Read the model definition and answer for the solid it produces. Units are mm, in the model's axes. Face numbers are marked on the shaded views. Coordinates: 2 decimals unless noted, no trailing zeros. Order: outer loops, then holes, each group sorted by start corner. A loop starts at its lowest first (then second) coordinate and runs counter-clockwise, first axis right, second up. Notation, with made-up numbers: (16.5, 84) -> (28.5, 84) arc R18 ccw to (28.5, 90) -> close; hole circle Ø6 at (-17, 89.5). An arc over 180 degrees is marked (long way). Answer in a Markdown table with one row per item.
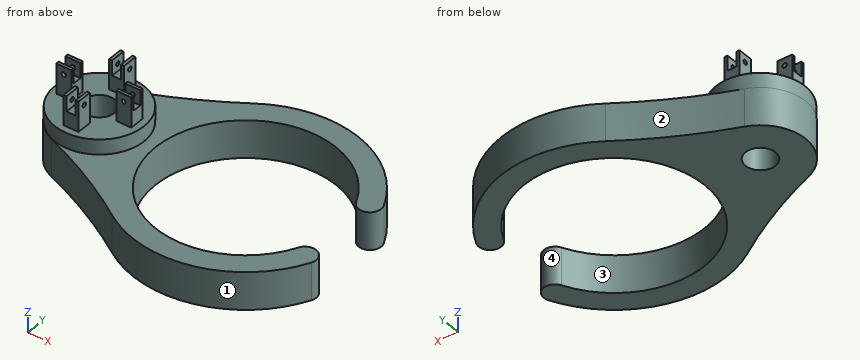
from build123d import *

# Parameters (mm, degrees)
BOSS_EXTRUDE1_DEPTH = 25
SKETCH1_3_R         = 29.652029199
BOSS_EXTRUDE2_DEPTH = 35
SKETCH3_R           = 10
CUT_EXTRUDE1_DEPTH  = 35
SKETCH4_W           = 10
SKETCH4_H           = 10
BOSS_EXTRUDE3_DEPTH = 20
SKETCH5_W           = 6
SKETCH5_H           = 10
SKETCH5_W_2         = 10
SKETCH5_H_2         = 6
CUT_EXTRUDE2_DEPTH  = 10
SKETCH6_R           = 1.3
SKETCH6_R_2         = 1.5
CUT_EXTRUDE3_DEPTH  = 10
SKETCH7_R           = 1.5
CUT_EXTRUDE4_DEPTH  = 10


with BuildPart() as part:
    # Sketch1 → Boss-Extrude1 (new body)
    with BuildSketch(Plane.XY):
        with BuildLine():
            ThreePointArc((50.600725893, 12.618751535), (112.455741461, 2.776716043), (160.210090254, 43.303630369))
            ThreePointArc((160.210090254, 43.303630369), (156.582418814, 53.270575735), (146.615473448, 49.642904296))
            ThreePointArc((146.615473448, 49.642904296), (32.237006226, 75), (146.615473448, 100.357095704))
            ThreePointArc((146.615473448, 100.357095704), (156.582418814, 96.729424265), (160.210090254, 106.696369631))
            ThreePointArc((160.210090254, 106.696369631), (112.455741461, 147.223283957), (50.600725893, 137.381248465))
            ThreePointArc((50.600725893, 137.381248465), (18.262261371, 118.334618782), (-16.010570265, 103.040064143))
            ThreePointArc((-16.010570265, 103.040064143), (-35.344980602, 75), (-16.010570265, 46.959935857))
            ThreePointArc((-16.010570265, 46.959935857), (18.262261371, 31.665381218), (50.600725893, 12.618751535))
        make_face()
    extrude(amount=BOSS_EXTRUDE1_DEPTH)

    # Sketch1<3> → Boss-Extrude2 (add)
    with BuildSketch(Plane.XY):
        with Locations((-5.344980602, 75)):
            Circle(SKETCH1_3_R)
    extrude(amount=BOSS_EXTRUDE2_DEPTH)

    # Sketch3 → Cut-Extrude1 (cut)
    with BuildSketch(Plane.XY.offset(35)):
        with Locations((-5.344980602, 75)):
            Circle(SKETCH3_R)
    extrude(amount=-CUT_EXTRUDE1_DEPTH, mode=Mode.SUBTRACT)

    # Sketch4 → Boss-Extrude3 (add)
    with BuildSketch(Plane.XY.offset(35)):
        with Locations((14.655019398, 75)):
            Rectangle(SKETCH4_W, SKETCH4_H)
        with Locations((-5.344980602, 55)):
            Rectangle(SKETCH4_W, SKETCH4_H)
        with Locations((-5.344980602, 95)):
            Rectangle(SKETCH4_W, SKETCH4_H)
        with Locations((-25.344980602, 75)):
            Rectangle(SKETCH4_W, SKETCH4_H)
    extrude(amount=BOSS_EXTRUDE3_DEPTH)

    # Sketch5 → Cut-Extrude2 (cut)
    with BuildSketch(Plane.XY.offset(55)):
        with Locations((-5.344980602, 95)):
            Rectangle(SKETCH5_W, SKETCH5_H)
        with Locations((14.655019398, 75)):
            Rectangle(SKETCH5_W_2, SKETCH5_H_2)
        with Locations((-5.344980602, 55)):
            Rectangle(SKETCH5_W, SKETCH5_H)
        with Locations((-25.344980602, 75)):
            Rectangle(SKETCH5_W_2, SKETCH5_H_2)
    extrude(amount=-CUT_EXTRUDE2_DEPTH, mode=Mode.SUBTRACT)

    # Sketch6 → Cut-Extrude3 (cut)
    with BuildSketch(Plane(origin=(0, 70, 0), x_dir=(-1, 0, 0), z_dir=(0, -1, 0))):
        with Locations(Location((-14.655019398, -50, 0), (0, 0, 180))):
            Circle(SKETCH6_R)
        with Locations(Location((25.344980602, -50, 0), (0, 0, 180))):
            Circle(SKETCH6_R_2)
    extrude(amount=-CUT_EXTRUDE3_DEPTH, mode=Mode.SUBTRACT)

    # Sketch7 → Cut-Extrude4 (cut)
    with BuildSketch(Plane.ZY.offset(10.344980602)):
        with Locations(Location((50, 55, 0), (0, 0, 270))):
            Circle(SKETCH7_R)
        with Locations(Location((50, 95, 0), (0, 0, 270))):
            Circle(SKETCH7_R)
    extrude(amount=-CUT_EXTRUDE4_DEPTH, mode=Mode.SUBTRACT)


solid = part.part
Q1. Consider line 1 (Z direction, x = -9.2, y = 95); line 2 (Z direction, x = 4, y = 108); line 3 (Y direction, x = 148.5, z = 11). Determine where each line is inside the solid, lowest interval first.
Outcome:
| item | result |
|---|---|
| line 1 | 0 to 48.5, 51.5 to 55 |
| line 2 | 0 to 25 |
| line 3 | 25.41 to 52.14, 97.86 to 124.59 |
Q2. The part is cut by section B-B (y = 75). Write down the section's boundary in (x, z).
Outcome:
| item | result |
|---|---|
| outline | (-35.34, 0) -> (-15.34, 0) -> (-15.34, 35) -> (-20.34, 35) -> (-20.34, 45) -> (-30.34, 45) -> (-30.34, 35) -> (-35, 35) -> (-35, 25) -> (-35.34, 25) -> close; (4.66, 0) -> (32.24, 0) -> (32.24, 25) -> (24.31, 25) -> (24.31, 35) -> (19.66, 35) -> (19.66, 45) -> (9.66, 45) -> (9.66, 35) -> (4.66, 35) -> close |
Q3. The part is cut by section A-A (z = 38). Write down the section's boundary in (x, y).
Outcome:
| item | result |
|---|---|
| outline | (-30.34, 70) -> (-20.34, 70) -> (-20.34, 80) -> (-30.34, 80) -> close; (-10.34, 50) -> (-0.34, 50) -> (-0.34, 60) -> (-10.34, 60) -> close; (-10.34, 90) -> (-0.34, 90) -> (-0.34, 100) -> (-10.34, 100) -> close; (9.66, 70) -> (19.66, 70) -> (19.66, 80) -> (9.66, 80) -> close |
Q4. The part is cut by section D-D (z = 17). Write down the section's boundary in (x, y).
Outcome:
| item | result |
|---|---|
| outline | (-16.01, 46.96) arc R333.67 cw to (50.6, 12.62) arc R75 ccw to (160.21, 43.3) arc R7.5 ccw to (146.62, 49.64) arc R60 cw (long way) to (146.62, 100.36) arc R7.5 ccw to (160.21, 106.7) arc R75 ccw to (50.6, 137.38) arc R333.67 cw to (-16.01, 103.04) arc R30 ccw to start; hole circle Ø20 at (-5.34, 75) |
Q5. Given pin 1 (6.5 mm diameter, centred on x = -6, y = 57, fed in from +Z); pin 2 (1.8 mm diameter, centred on x = -23, y = 75.5, fed in from +Z); pin 3 (5 mm diameter, centred on y = 95, z = 7, fed in from -X); pin 4 (5 mm diameter, centred on y = 95, z = 50, fed in from -X) (3 decimals), each flat-ended and moving along its own axis, determine where each tip first touches the part or whether it passes through.
Outcome:
| item | result |
|---|---|
| pin 1 | z = 55 |
| pin 2 | z = 45 |
| pin 3 | x = -29.71 |
| pin 4 | x = -10.345 |
Q6. The part is cut by section C-C (x = 91). Write down the section's boundary in (y, z), then the cut area to 3 significant figures.
Outcome:
| item | result |
|---|---|
| outline | (0.01, 0) -> (15.01, 0) -> (15.01, 25) -> (0.01, 25) -> close; (134.99, 0) -> (149.99, 0) -> (149.99, 25) -> (134.99, 25) -> close |
| area | 750 mm² |
Q7. For a pull along Y with two mould halves and no side action, classify the marked faces 1, 2, 3 and 4 as pulls with the +Y half, pulls with the -Y half, needs draft (parallel to the pull), parting line crosses it, or undercut.
Outcome:
| item | result |
|---|---|
| face 1 | pulls with the -Y half |
| face 2 | pulls with the +Y half |
| face 3 | undercut |
| face 4 | undercut |
